Answer from the drawing. Dimensions are ordinates in mm from the lowest x, y and z of the part. Give positions to 0.01 mm unless a question says otherwise; leave off trailing zeros. Loops run counter-clockwise (first coordinate to the right, second up) from the corner with the lowest first, then second, coordinate; pieces in that order, holes last. Notation, with made-up numbers: (-22, 24) -> (3, 24) arc R16 ccw to (3, 37) -> close; hole circle Ø5 at (-14, 43.5). An arc over 180 degrees is marked (long way). Answer as CSV lines item,"result". Start each with the question number.
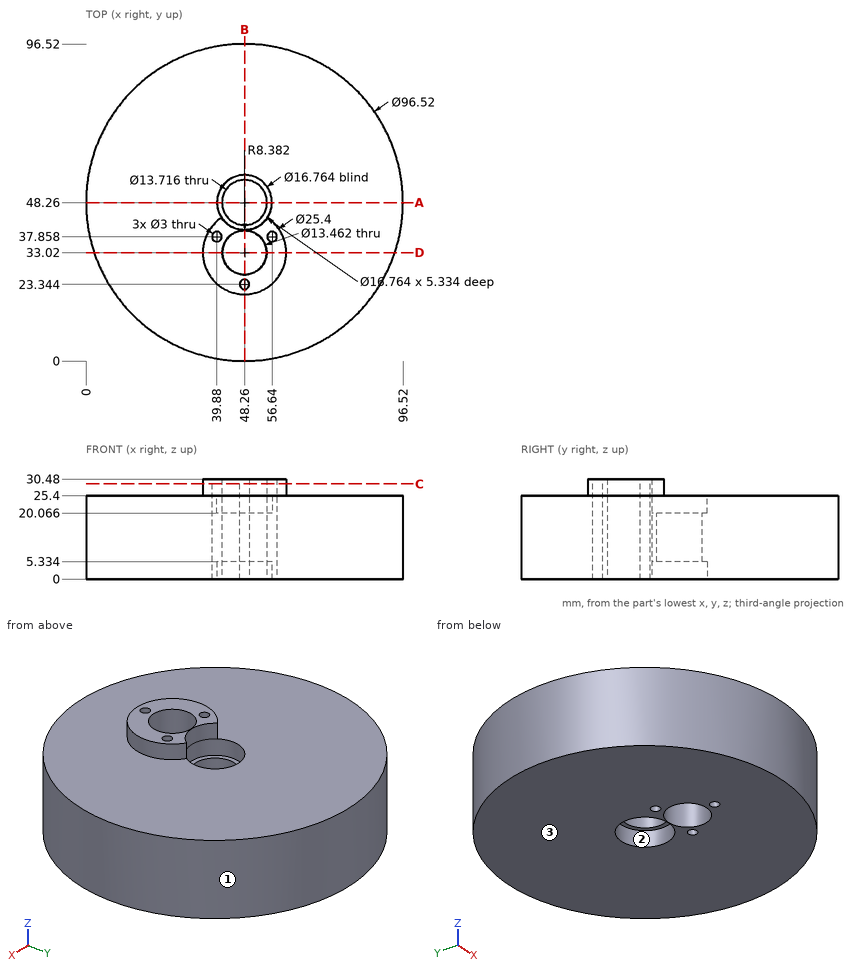
(1) Find section D-D on y = 33.02. Write down the section's boundary in (x, z).
(2) Find section C-C on z = 29. Write down the section's boundary in (x, y) (1 decimal).
(3) The mould has two halves that part along Y. Classify the marked faces 1, 2 and 3: pulls with the +Y half, pulls with the -Y half, needs draft (parallel to the pull), parting line crosses it, or undercut.
(4) Find section A-A on y = 48.26. Write down the section's boundary in (x, z).
(5) Find section B-B on x = 48.26. Write down the section's boundary in (y, z).
(6) Each of these flat-tipped pins is pushed along its axis until it touches: P1, Ø13.5, axis at x = 48.26, y = 48.26, coming from the -Z side; P2, Ø3, axis at x = 42.5, y = 67.5, coming from the +Z side; P3, Ø1.5, axis at x = 60, z = 12.5, coming from the +Y side; P4, Ø1, axis at x = 61.5, z = 19.5, coming from the +Y side. Where does it stop, or does it pass through?
(7) Find the intervals of material crossed by line 1 along Y through (x, z) = (48.26, 12); line 2 along Y through (x, z) = (48, 16); line 3 along Z through (x, y) = (14, 50), in increasing order. Write a range as from..to.
Answer block:
1,outline,"(2.47, 0) -> (41.53, 0) -> (41.53, 30.48) -> (35.56, 30.48) -> (35.56, 25.4) -> (2.47, 25.4) -> close; (54.99, 0) -> (94.05, 0) -> (94.05, 25.4) -> (60.96, 25.4) -> (60.96, 30.48) -> (54.99, 30.48) -> close"
2,outline,"(41.3, 43.6) arc R12.7 ccw (long way) to (55.2, 43.6) arc R8.4 cw to start; hole circle Ø3 at (39.9, 37.9); hole circle Ø13.5 at (48.3, 33); hole circle Ø3 at (48.3, 23.3); hole circle Ø3 at (56.6, 37.9)"
3,face 1,"parting line crosses it"
3,face 2,"undercut"
3,face 3,"needs draft"
4,outline,"(0, 0) -> (39.88, 0) -> (39.88, 5.33) -> (41.4, 5.33) -> (41.4, 20.07) -> (39.88, 20.07) -> (39.88, 25.4) -> (0, 25.4) -> close; (55.12, 5.33) -> (56.64, 5.33) -> (56.64, 0) -> (96.52, 0) -> (96.52, 25.4) -> (56.64, 25.4) -> (56.64, 20.07) -> (55.12, 20.07) -> close"
5,outline,"(0, 0) -> (21.84, 0) -> (21.84, 30.48) -> (20.32, 30.48) -> (20.32, 25.4) -> (0, 25.4) -> close; (24.84, 0) -> (26.29, 0) -> (26.29, 30.48) -> (24.84, 30.48) -> close; (39.75, 0) -> (39.88, 0) -> (39.88, 5.33) -> (41.4, 5.33) -> (41.4, 20.07) -> (39.88, 20.07) -> (39.88, 30.48) -> (39.75, 30.48) -> close; (55.12, 5.33) -> (56.64, 5.33) -> (56.64, 0) -> (96.52, 0) -> (96.52, 25.4) -> (56.64, 25.4) -> (56.64, 20.07) -> (55.12, 20.07) -> close"
6,P1,"passes through"
6,P2,"stops at z = 25.4"
6,P3,"stops at y = 95.25"
6,P4,"stops at y = 94.81"
7,line 1,"y = 0..21.84, 24.84..26.29, 39.75..41.4, 55.12..96.52"
7,line 2,"y = 0..21.87, 24.82..26.29, 39.75..41.41, 55.11..96.52"
7,line 3,"z = 0..25.4"
